Part model, mm, in its own coordinate system. A direction names the side the tool comes from. Round coordinates to 2 decimals unless told otherwise and drop trailing zeros. Write each loop counter-clockwise with the first axis right and the second up, starting at its lowest first coordinate (ties: lowest second). Pieces come first, ordered by that corner, then holes. Notation, with made-up numbers: M -21.75,-15.5 L -3.75,-15.5 A23 ccw -3.75,-1.5 Z; hole C 0.25,-17.75 d3. An arc over 180 degrees is marked long. Use one line per item in the form item = value. Start each with the question number.
Item 1: Flat gauge pins, fed straight in: pin 1 Ø5 at (x, z) = (-5.5, 26) entering from +Y; pin 2 Ø3 at (x, y) = (24.5, 22.5) entering from -Z; pin 3 Ø8.5 at (y, z) = (13, 14.5) entering from +X. Where does each tip first touch, or does it go through?
Item 2: Mould opens along X. For faces 5 (the face through (17.923, 30.086, 40.846)), 6 (the face through (1, 15, 52)), 7 (the face through (-0.33, 29.504, 25.636)), 8 (the face through (-4.5, 13, 26)) say: +X half, -X half, draft (parallel to the pull), parting line (faces both ways), or undercut.
Item 3: Cut at B-B, the plane x = -22. Give the cut face in (y, z), then the cut area to 3 significant figures.
Item 4: Which spindle directions (+Z, -Z, +X, -X, +Y, -Y) get a long thin tool onto all of the face, cutting with end or side? Do faces 1 (the face through (-17.64, 29.74, 25.64)), 2 (the face through (-19, 44.5, 26)), 3 (the face through (21, 16, 30)), 4 (the face through (13.88, 33.38, 10.85)). Say none if no direction does.
Item 5: Cut at C-C, the plane y = 15. Give the cut face in (x, z).
Item 6: Cut at A-A, the plane z = 6.5. Give the cut face in (x, y), then the cut area to 3 significant figures.
Item 7: Probe L1, parallel to X at y = 13, z = 45; L2, parallel to Z at x = 17.5, y = 7. List the from-to ranges inside material, lowest first.
Item 8: Cut at D-D, the plane x = 28.5. Give the cut face in (y, z), then the cut area to 3 significant figures.
from build123d import *

# Parameters (mm, degrees)
BOSS_EXTRUDE3_DEPTH = 52
BOSS_EXTRUDE4_DEPTH = 30
CUT_EXTRUDE1_DEPTH  = 22


with BuildPart() as part:
    # Sketch4 → Boss-Extrude3 (new body)
    with BuildSketch(Plane.XY):
        with BuildLine():
            Line((-37.5, 4.5), (-4.5, 4.5))
            Line((-4.5, 4.5), (-4.5, 21.944512863))
            ThreePointArc((-4.5, 21.944512863), (-17.783419244, 29.914047854), (-23, 44.5))
            Line((-23, 44.5), (-15, 44.5))
            ThreePointArc((-15, 44.5), (0, 29.5), (15, 44.5))
            Line((15, 44.5), (23, 44.5))
            ThreePointArc((23, 44.5), (17.783419244, 29.914047854), (4.5, 21.944512863))
            Line((4.5, 21.944512863), (4.5, 4.5))
            Line((4.5, 4.5), (37.5, 4.5))
            Line((37.5, 4.5), (37.5, -4.5))
            Line((37.5, -4.5), (-37.5, -4.5))
            Line((-37.5, -4.5), (-37.5, 4.5))
        make_face()
    extrude(amount=BOSS_EXTRUDE3_DEPTH)

    # Sketch5 → Boss-Extrude4 (add)
    with BuildSketch(Plane.XY):
        Polygon((4.5, 4.5), (37.5, 4.5), (23, 44.5), (4.5, 21.944512863), align=None)
    extrude(amount=BOSS_EXTRUDE4_DEPTH)

    # Sketch5<2> → Cut-Extrude1 (cut)
    with BuildSketch(Plane.XY):
        Polygon((4.5, 4.5), (37.5, 4.5), (23, 44.5), (4.5, 21.944512863), align=None)
    extrude(amount=CUT_EXTRUDE1_DEPTH, mode=Mode.SUBTRACT)


solid = part.part
Model answer:
q1.pin_1 = 31.81
q1.pin_2 = 22
q1.pin_3 = 4.5
q2.face_5 = +X half
q2.face_6 = draft
q2.face_7 = undercut
q2.face_8 = -X half
q3.outline = M -4.5,0 L 4.5,0 L 4.5,52 L -4.5,52 Z; M 37.79,0 L 44.5,0 L 44.5,52 L 37.79,52 Z
q3.area = 817 mm²
q4.face_1 = +Z, -Z, -X
q4.face_2 = +Z, -Z, +X, -X, +Y
q4.face_3 = +Z, +X
q4.face_4 = -Z, +X
q5.outline = M -4.5,0 L 4.5,0 L 4.5,22 L 33.69,22 L 33.69,30 L 4.5,30 L 4.5,52 L -4.5,52 Z
q6.outline = M -37.5,-4.5 L 37.5,-4.5 L 37.5,4.5 L 4.5,4.5 L 4.5,21.94 L 23,44.5 L 15,44.5 A15 cw -15,44.5 L -23,44.5 A23 ccw -4.5,21.94 L -4.5,4.5 L -37.5,4.5 Z
q6.area = 1,200 mm²
q7.L1 = -4.5 to 4.5
q7.L2 = 22 to 30
q8.outline = M -4.5,0 L 4.5,0 L 4.5,22 L 29.33,22 L 29.33,30 L 4.5,30 L 4.5,52 L -4.5,52 Z
q8.area = 667 mm²
